Here's how the part is built. I have some questions about the finished solid (model axes, mm). A direction names the side the tool comes from. Coordinates: 2 decimals unless noted, no trailing zeros. Write each loop counter-clockwise with the first axis right and the second up, starting at its lowest first coordinate (ties: lowest second). Pieces come first, ordered by that corner, then holes. Notation, with made-up numbers: M 67,18.25 L 76,18.25 A14 cw 76,23.25 Z; hole C 36,3.25 d9. An arc over 180 degrees is marked long. Use a Markdown table: item, result.
```python
from build123d import *

# Parameters (mm, degrees)
EXTRUDE_1_DEPTH                = 4
EXTRUDE_2_DEPTH                = 1
HOLE_WIZARD_M5_1_D             = 5.5
HOLE_WIZARD_M5_1_CSINK_D       = 5.55
HOLE_WIZARD_M5_1_CSINK_ANGLE   = 90
EXTRUDE_START                  = -4
EXTRUDE_3_DEPTH                = 6.5
SKETCH_22_W                    = 52.393711498
SKETCH_22_H                    = 4
EXTRUDE_4_DEPTH                = 4
SKETCH_23_R                    = 4
EXTRUDE_5_DEPTH                = 5
HOLE_WIZARD_M2_5_1_D           = 2.9
HOLE_WIZARD_M2_5_1_DEPTH       = 10
HOLE_WIZARD_M2_5_1_CSINK_D     = 2.95
HOLE_WIZARD_M2_5_1_CSINK_ANGLE = 90
HOLE_WIZARD_M2_5_1_TIP         = 0.871247898
SKETCH_27_R                    = 2.5
CUT_EXTRUDE_4_DEPTH            = 5
SKETCH_28_R                    = 5
EXTRUDE_6_DEPTH                = 1
SKETCH_29_R                    = 4.5
EXTRUDE_7_DEPTH                = 6
SKETCH_30_R                    = 4.5
EXTRUDE_8_DEPTH                = 4
HOLE_WIZARD_M5_1_2_D           = 4.2
HOLE_WIZARD_M5_1_2_CSINK_D     = 4.25
HOLE_WIZARD_M5_1_2_CSINK_ANGLE = 90
HOLE_WIZARD_M5_2_D             = 5.5
HOLE_WIZARD_M5_2_DEPTH         = 10
HOLE_WIZARD_M5_2_CSINK_D       = 5.55
HOLE_WIZARD_M5_2_CSINK_ANGLE   = 90
HOLE_WIZARD_M5_2_TIP           = 1.652366702


with BuildPart() as part:
    # 草图2 → 凸台-拉伸1 (new body)
    with BuildSketch(Plane.XY):
        Polygon((80, 0), (-80, 0), (-120, 60), (-105, 70), (105, 70), (120, 60), align=None)
    extrude(amount=EXTRUDE_1_DEPTH)

    # 草图3 → 凸台-拉伸2 (add)
    with BuildSketch(Plane.XY.offset(4)):
        Polygon((105, 70), (99, 70), (99, 55), (100, 55), (100, 48), (99, 48), (99, 40), (106.666666667, 40), (120, 60), align=None)
        Polygon((-120, 60), (-105, 70), (-99, 70), (-99, 55), (-100, 55), (-100, 48), (-99, 48), (-99, 40), (-106.666666667, 40), align=None)
    extrude(amount=EXTRUDE_2_DEPTH)

    # Hole Wizard M5 _1 (through all)
    with Locations(Plane.XY.offset(5)):
        with Locations((-109, 59.5), (109, 59.5)):
            CounterSinkHole(HOLE_WIZARD_M5_1_D / 2, HOLE_WIZARD_M5_1_CSINK_D / 2, counter_sink_angle=HOLE_WIZARD_M5_1_CSINK_ANGLE)

    # 草图21 → 凸台-拉伸3 (add)
    with BuildSketch(Plane.XY.offset(4).offset(EXTRUDE_START)):
        Polygon((-70, 0), (-45, -4), (-30, -4), (-12.5, -8), (12.5, -8), (30, -4), (45, -4), (70, 0), (80, 0), (82.666666667, 4), (70, 4), (45, 0), (26.196855749, 0), (26.196855749, -4), (-26.196855749, -4), (-26.196855749, 0), (-45, 0), (-70, 4), (-82.666666667, 4), (-80, 0), align=None)
    extrude(amount=EXTRUDE_3_DEPTH)

    # 草图22 → 凸台-拉伸4 (add)
    with BuildSketch(Plane.XZ):
        with Locations((0, 2)):
            Rectangle(SKETCH_22_W, SKETCH_22_H)
    extrude(amount=EXTRUDE_4_DEPTH)

    # 草图23 → 凸台-拉伸5 (add)
    with BuildSketch(Plane.XY.offset(6.5)):
        with Locations((-75, 0)):
            Circle(SKETCH_23_R)
        with Locations((-37.5, -4)):
            Circle(SKETCH_23_R)
        with Locations((37.5, -4)):
            Circle(SKETCH_23_R)
        with Locations((75, 0)):
            Circle(SKETCH_23_R)
    extrude(amount=-EXTRUDE_5_DEPTH)

    # M2.5 间隙孔1
    with Locations(Plane(origin=(0, 0, 0), x_dir=(-1, 0, 0), z_dir=(0, 0, -1))):
        with Locations((-75, 0), (-37.5, -4), (37.5, -4), (75, 0)):
            CounterSinkHole(HOLE_WIZARD_M2_5_1_D / 2, HOLE_WIZARD_M2_5_1_CSINK_D / 2, depth=HOLE_WIZARD_M2_5_1_DEPTH, counter_sink_angle=HOLE_WIZARD_M2_5_1_CSINK_ANGLE)
            with Locations((0, 0, -(HOLE_WIZARD_M2_5_1_DEPTH + HOLE_WIZARD_M2_5_1_TIP / 2))):  # 118° drill point
                Cone(0, HOLE_WIZARD_M2_5_1_D / 2, HOLE_WIZARD_M2_5_1_TIP, mode=Mode.SUBTRACT)

    # 草图27 → 切除-拉伸4 (cut)
    with BuildSketch(Plane(origin=(0, 0, 0), x_dir=(-1, 0, 0), z_dir=(0, 0, -1))):
        with Locations((-75, 0)):
            Circle(SKETCH_27_R)
        with Locations((-37.5, -4)):
            Circle(SKETCH_27_R)
        with Locations((75, 0)):
            Circle(SKETCH_27_R)
        with Locations((37.5, -4)):
            Circle(SKETCH_27_R)
    extrude(amount=-CUT_EXTRUDE_4_DEPTH, mode=Mode.SUBTRACT)

    # 草图28 → 凸台-拉伸6 (add)
    with BuildSketch(Plane.XY.offset(4)):
        with Locations(Location((-20, 14.25, 0), (0, 0, 180))):
            Circle(SKETCH_28_R)
        with Locations(Location((-29, 36, 0), (0, 0, 180))):
            Circle(SKETCH_28_R)
        with Locations(Location((-11, 36, 0), (0, 0, 180))):
            Circle(SKETCH_28_R)
    extrude(amount=EXTRUDE_6_DEPTH)

    # 草图29 → 凸台-拉伸7 (add)
    with BuildSketch(Plane.XY.offset(5)):
        with Locations((-20, 14.25)):
            Circle(SKETCH_29_R)
    extrude(amount=EXTRUDE_7_DEPTH)

    # 草图30 → 凸台-拉伸8 (add)
    with BuildSketch(Plane.XY.offset(5)):
        with Locations((-11, 36)):
            Circle(SKETCH_30_R)
        with Locations((-29, 36)):
            Circle(SKETCH_30_R)
    extrude(amount=EXTRUDE_8_DEPTH)

    # Hole Wizard M5 _1 2 (through all)
    with Locations(Plane.XY.offset(9)):
        with Locations((-29, 36), (-11, 36)):
            CounterSinkHole(HOLE_WIZARD_M5_1_2_D / 2, HOLE_WIZARD_M5_1_2_CSINK_D / 2, counter_sink_angle=HOLE_WIZARD_M5_1_2_CSINK_ANGLE)

    # M5 间隙孔2
    with Locations(Plane.XY.offset(4)):
        with Locations((-96.286602224, 31.641005887), (-85.192598299, 15), (96.286602224, 31.641005887), (85.192598299, 15)):
            CounterSinkHole(HOLE_WIZARD_M5_2_D / 2, HOLE_WIZARD_M5_2_CSINK_D / 2, depth=HOLE_WIZARD_M5_2_DEPTH, counter_sink_angle=HOLE_WIZARD_M5_2_CSINK_ANGLE)
            with Locations((0, 0, -(HOLE_WIZARD_M5_2_DEPTH + HOLE_WIZARD_M5_2_TIP / 2))):  # 118° drill point
                Cone(0, HOLE_WIZARD_M5_2_D / 2, HOLE_WIZARD_M5_2_TIP, mode=Mode.SUBTRACT)


solid = part.part
```
1. We'd pull the mould along X, two halves only. Please class faces 1 (the face through (-39, -5, 5)), 2 (the face through (-18.92, 19.13, 4.49)), 3 (the face through (37, -7, 1.5)): +X half, -X half, draft (parallel to the pull), parting line (faces both ways), or undercut.
Answers follow:
| item | result |
|---|---|
| face 1 | undercut |
| face 2 | parting line |
| face 3 | draft |
2. I need wall thicknesses on probe 1 along X at (y, z) = (59.5, 3.5); probe 2 along X at (y, z) = (15, 3); probe 3 along Y at (x, z) = (-37.5, 5.95). Which ranges of each line are inside material? Lowest first, please.
Answers follow:
| item | result |
|---|---|
| probe 1 | x = -119.67 to -111.75, -106.25 to 106.25, 111.75 to 119.67 |
| probe 2 | x = -90 to -87.94, -82.44 to 82.44, 87.94 to 90 |
| probe 3 | y = -8 to -5.45, -2.55 to 0 |
3. Will these pins go through, and if not, where does the flat tip stop? pin 1 Ø2 at (x, y) = (-32, 35.5) entering from -Z; pin 2 Ø0.8 at (x, z) = (-102, 4.5) entering from -Y; pin 3 Ø4 at (x, y) = (-37.5, -4) entering from +Z; pin 4 Ø1.5 at (x, z) = (63, 4.5) entering from -Y.
Answers follow:
| item | result |
|---|---|
| pin 1 | stops at z = 0 |
| pin 2 | stops at y = 40 |
| pin 3 | stops at z = 6.5 |
| pin 4 | stops at y = -1.24 |
4. Suppose I cut it at A-A on x = -52. Write out the boundary of the cut face in (y, z), and give its area (3 significant figures).
Answers follow:
| item | result |
|---|---|
| outline | M -2.88,0 L 70,0 L 70,4 L 1.12,4 L 1.12,6.5 L -2.88,6.5 Z |
| area | 302 mm2 |
5. Suppose I cut it at B-B on y = 21.5. Write out the boundary of the cut face in (x, z).
Answers follow:
| item | result |
|---|---|
| outline | M -94.33,0 L 94.33,0 L 94.33,4 L -94.33,4 Z |
6. Which directions (+Z, -Z, +X, -X, +Y, -Y) give clear straight access to the entire face, cutting with the end or side of a thin tool? Please do faces 4 (the face through (-11.98, 31.61, 6.97)), 5 (the face through (-38, -7, 1.5)), 6 (the face through (75, -2, 5)).
Answers follow:
| item | result |
|---|---|
| face 4 | +Z |
| face 5 | -Z, -X, -Y |
| face 6 | -Z |
